Part model, mm, in its own coordinate system. Face numbers are marked on the shaded views. A direction names the side the tool comes from. Coordinates: 2 decimals unless noted, no trailing zeros. Loops run counter-clockwise (first coordinate to the right, second up) from the corner with the lowest first, then second, coordinate; pieces in that order, holes last. Notation, with made-up numbers: (74.25, -19.5) - (89.25, -19.5) arc R16 cw to (89.25, 8.5) - close; hole circle Ø5 at (-10, 34.5). An arc over 180 degrees is marked (long way). Use a Markdown table: item, result. Add a question column.
1) Drop flat-ended pins along their axis: P1, Ø12, axis at x = 8, z = -26.5, coming from the +Y side; P2, Ø1.5, axis at x = -8, y = 17, coming from the +Z side; P3, Ø3, axis at x = 0, z = 28, coming from the -Y side; P4, Ø1, axis at x = -0.5, y = 11, coming from the +Z side. Give the stop position or say it passes through.
2) Band-saw the part on C-C (x = 7.75). Give the cut face in (y, z).
3) Band-saw the part on A-A (x = 0). Give the cut face in (y, z).
4) Probe probe 1 along Z at (x, y) = (0, 3.5); probe 2 along X at (y, z) = (3.25, -28); probe 3 along Y at (x, z) = (0.25, -30.5). List the from-to ranges inside material, lowest first. Write a range as [from, to].
5) Tool access for the marked faces 1, 2 and 3: list every direction of +Z, -Z, +X, -X, +Y, -Y with a clear straight run to the whole face (end or side of a thin tool).
6) Band-saw the part on B-B (z = 28). Give the cut face in (x, y), plus the area to 3 significant figures.
7) Band-saw the part on D-D (y = 21.25). Give the cut face in (x, z), plus the area to 3 significant figures.
Autodesk Inventor part; units mm, degrees
ref_plane "YZ Plane" through (0, 0, 0) normal (1, 0, 0) x (0, 1, 0)
ref_plane "XZ Plane" through (0, 0, 0) normal (0, 1, 0) x (-1, 0, 0)
ref_plane "XY Plane" through (0, 0, 0) normal (0, 0, 1) x (1, 0, 0)
sketch "Sketch1" plane through (0, 0, 0) normal (0, 1, 0) x (-1, 0, 0)
  line L0 (11, 36) -> (-11, 36)
  line L1 (-11, 36) -> (-11, -36)
  line L2 (-11, -36) -> (11, -36)
  line L3 (11, -36) -> (11, 36)
  line L4 (11, 36) -> (-11, -36) construction
  line L5 (-11, 36) -> (11, -36) construction
  point P0 (0, 0)
extrude "Extrusion1" add sketch "Sketch1" along normal blind 10
sketch "Sketch2" plane through (0, 10, 0) normal (0, 1, 0) x (1, 0, 0)
  point P0 (0, 0)
  point P1 (0, -28)
  point P2 (0, 28)
hole "Hole1" at (0, 10, 28) at (0, 10, -28) direction (0, -1, 0) diameter 3.242 depth 10
sketch "Sketch3" plane through (0, 10, 0) normal (0, 1, 0) x (1, 0, 0)
  line L0 (11, -36) -> (11, 36)
  line L1 (-11, -20) -> (11, -20)
  line L2 (11, -20) -> (11, 20)
  line L3 (11, 20) -> (-11, 20)
  line L4 (-11, 20) -> (-11, -20)
  line L5 (-11, -20) -> (11, 20) construction
  line L6 (11, -20) -> (-11, 20) construction
  point P0 (0, 0)
extrude "Extrusion2" add sketch "Sketch3" along normal blind 18
chamfer "Chamfer1" distance 16 angle 45 2 edges at (0, 28, -20) (0, 28, 20)
fillet "Fillet1" radius 4 2 edges at (0, 28, 4) (0, 28, -4)
sketch "Sketch4" plane through (-11, 12, 20) normal (0, 0.7071, 0.7071) x (1, 0, 0)
  point P0 (11, 5.6569)
  point P1 (11, 12)
sketch "Sketch5" plane through (11, 12, -20) normal (0, 0.7071, -0.7071) x (-1, 0, 0)
  point P0 (11, 5.6569)
  point P1 (11, 12)
properties part number "StrutConnector"
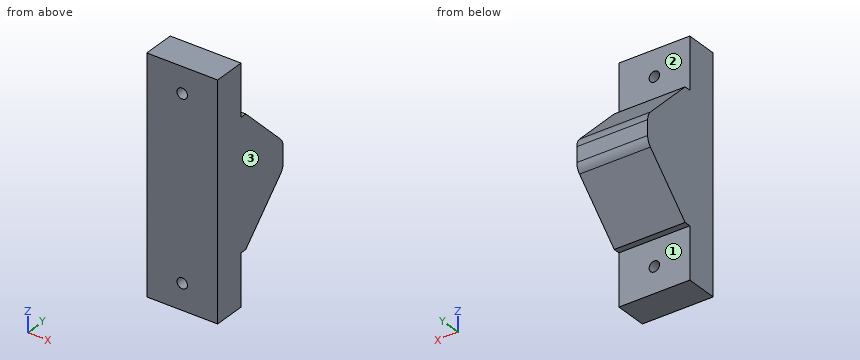
Answer block:
| question | item | result |
|---|---|---|
| 1 | P1 | y = 10 |
| 1 | P2 | z = 15.75 |
| 1 | P3 | through |
| 1 | P4 | z = 20 |
| 2 | outline | (0, -36) - (10, -36) - (10, -20) - (12, -20) - (26.83, -5.17) arc R4 ccw to (28, -2.34) - (28, 2.34) arc R4 ccw to (26.83, 5.17) - (12, 20) - (10, 20) - (10, 36) - (0, 36) - close |
| 3 | outline | (0, -36) - (10, -36) - (10, -29.62) - (0, -29.62) - close; (0, -26.38) - (10, -26.38) - (10, -20) - (12, -20) - (26.83, -5.17) arc R4 ccw to (28, -2.34) - (28, 2.34) arc R4 ccw to (26.83, 5.17) - (12, 20) - (10, 20) - (10, 26.38) - (0, 26.38) - close; (0, 29.62) - (10, 29.62) - (10, 36) - (0, 36) - close |
| 4 | probe 1 | [-36, -29.62], [-26.38, 26.38], [29.62, 36] |
| 4 | probe 2 | [-11, -1.62], [1.62, 11] |
| 4 | probe 3 | [0, 10] |
| 5 | face 1 | -Z, +X, -X, +Y |
| 5 | face 2 | +Z, +X, -X, +Y |
| 5 | face 3 | +Z, -Z, +X, +Y, -Y |
| 6 | outline | (-11, 0) - (-1.62, 0) - (-1.62, 10) - (-11, 10) - close; (1.62, 0) - (11, 0) - (11, 10) - (1.62, 10) - close |
| 6 | area | 188 mm2 |
| 7 | outline | (-11, -10.75) - (11, -10.75) - (11, 10.75) - (-11, 10.75) - close |
| 7 | area | 473 mm2 |
